Read the model definition and answer for the solid it produces. Units are mm, in the model's axes. A direction names the side the tool comes from. Coordinates: 2 decimals unless noted, no trailing zeros. Order: outer loops, then holes, each group sorted by start corner. A loop starts at its lowest first (then second) coordinate and runs counter-clockwise, first axis right, second up. Notation, with made-up numbers: (49, -10.5) - (69, -10.5) arc R22 ccw to (69, 14.5) - close; hole circle Ø2 at (-37.75, 1). An arc over 180 degrees is marked (long way). Use one line per item in the form item = value.
```python
from build123d import *

# Parameters (mm, degrees)
CROQUIS1_R              = 5
CROQUIS1_R_2            = 4.25
SALIENTE_EXTRUIR1_DEPTH = 19.6
CROQUIS2_R              = 9
CROQUIS2_R_2            = 4.25
SALIENTE_EXTRUIR2_DEPTH = 2
CROQUIS3_R              = 5
SALIENTE_EXTRUIR3_DEPTH = 5
CROQUIS4_R              = 2.25
CORTAR_EXTRUIR1_DEPTH   = 6
SALIENTE_EXTRUIR4_START = -16.6
CROQUIS5_R              = 4.25
SALIENTE_EXTRUIR4_DEPTH = 16.6


with BuildPart() as part:
    # Croquis1 → Saliente-Extruir1 (new body)
    with BuildSketch(Plane.XY):
        Circle(CROQUIS1_R)
        Circle(CROQUIS1_R_2, mode=Mode.SUBTRACT)
    extrude(amount=-SALIENTE_EXTRUIR1_DEPTH)

    # Croquis2 → Saliente-Extruir2 (add)
    with BuildSketch(Plane(origin=(0, 0, -19.6), x_dir=(-1, 0, 0), z_dir=(0, 0, -1))):
        Circle(CROQUIS2_R)
        with Locations(Location((0, 0, 0), (0, 0, 180))):
            Circle(CROQUIS2_R_2, mode=Mode.SUBTRACT)
    extrude(amount=SALIENTE_EXTRUIR2_DEPTH)

    # Croquis3 → Saliente-Extruir3 (add)
    with BuildSketch(Plane.XY):
        Circle(CROQUIS3_R)
    extrude(amount=-SALIENTE_EXTRUIR3_DEPTH)

    # Croquis4 → Cortar-Extruir1 (cut)
    with BuildSketch(Plane.XY):
        Circle(CROQUIS4_R)
    extrude(amount=-CORTAR_EXTRUIR1_DEPTH, mode=Mode.SUBTRACT)

    # Croquis5 → Saliente-Extruir4 (add)
    with BuildSketch(Plane(origin=(0, 0, -21.6), x_dir=(-1, 0, 0), z_dir=(0, 0, -1)).offset(SALIENTE_EXTRUIR4_START)):
        Circle(CROQUIS5_R)
    extrude(amount=SALIENTE_EXTRUIR4_DEPTH)


solid = part.part
```
(1) Given pin 1 Ø3 at (y, z) = (-1, -4.5) entering from -X; pin 2 Ø5 at (y, z) = (-2, -19) entering from +X; pin 3 Ø8 at (x, z) = (-5.5, -13) entering from -Y; pin 4 Ø3 at (x, y) = (-6.5, 4.5) entering from +Z, each flat-ended and moving along its own axis, determine where each tip first touches the part or whether it passes through.
Answer list:
pin_1 = -5
pin_2 = 9
pin_3 = -4.77
pin_4 = -19.6
(2) Straight lines are drawn through the part: L1, parallel to Y at x = 0, z = -3.55; L2, parallel to Z at x = 5, y = -4; L3, parallel to Y at x = 0, z = -18.75. For each, find the intervals that lie inside material, in ascending order.
Answer list:
L1 = -5 to -2.25, 2.25 to 5
L2 = -21.6 to -19.6
L3 = -5 to 5
(3) Section D-D, the plane z = -7 is taken. Write down the section's boundary in (x, y), then the cut area to 3 significant figures.
Answer list:
outline = circle Ø10 at (0, 0)
area = 78.5 mm2
(4) The mould has two halves that part along Y. Classify faces 3 (the cylindrical face through (-1.08, -4.88, -9.66)), 4 (the flat face through (-4, -4, -19.6)), 5 (the cylindrical face through (-0.29, 2.23, -2.46)): +Y half, -Y half, draft (parallel to the pull), parting line (faces both ways), or undercut.
Answer list:
face_3 = parting line
face_4 = draft
face_5 = undercut
(5) Which of the six approach directions +Z, -Z, +X, -X, +Y, -Y give full straight-line access (tool end or side, diameter ignored) to faces 1 (the flat face through (2.2, -1, 0)), 2 (the flat face through (0, 0, -5))?
Answer list:
face_1 = +Z, +X, -X, +Y, -Y
face_2 = +Z
(6) Section C-C, the plane z = -3.5 is taken. Write down the section's boundary in (x, y).
Answer list:
outline = circle Ø10 at (0, 0); hole circle Ø4.5 at (0, 0)
(7) Section A-A, the plane x = 0 is taken. Write down the section's boundary in (y, z).
Answer list:
outline = (-9, -21.6) - (9, -21.6) - (9, -19.6) - (5, -19.6) - (5, 0) - (2.25, 0) - (2.25, -5) - (-2.25, -5) - (-2.25, 0) - (-5, 0) - (-5, -19.6) - (-9, -19.6) - close
